from build123d import *

# Parameters (mm, degrees)
SKETCH_R    = 1.6
SKETCH_R_2  = 2.6
PAD_DEPTH   = 3
FILLET_R    = 3
FILLET001_R = 3
FILLET002_R = 3
FILLET003_R = 3
FILLET004_R = 3


with BuildPart() as part:
    # Sketch → Pad (new body)
    with BuildSketch(Plane.XY):
        Polygon((3, 50), (13, 50), (13, 37), (20, 37), (20, 23), (13, 23), (13, -20), (3, -20), (3, -7), (-4, -7), (-4, 7), (3, 7), align=None)
        Circle(SKETCH_R, mode=Mode.SUBTRACT)
        with Locations((16, 30)):
            Circle(SKETCH_R, mode=Mode.SUBTRACT)
        with Locations((8, 45)):
            Circle(SKETCH_R_2, mode=Mode.SUBTRACT)
        with Locations((8, -15)):
            Circle(SKETCH_R_2, mode=Mode.SUBTRACT)
    extrude(amount=PAD_DEPTH)

    # Fillet
    fillet_edges = [part.edges().sort_by_distance(p)[0] for p in [
        (13, -20, 1.5),
        (3, -20, 1.5),
        (20, 23, 1.5),
        (20, 37, 1.5),
        (-4, -7, 1.5),
        (-4, 7, 1.5),
        (3, 50, 1.5),
        (13, 50, 1.5),
    ]]
    fillet(fillet_edges, radius=FILLET_R)

    # Fillet001
    fillet001_edges = [part.edges().sort_by_distance(p)[0] for p in [
        (13, 37, 1.5),
    ]]
    fillet(fillet001_edges, radius=FILLET001_R)

    # Fillet002
    fillet002_edges = [part.edges().sort_by_distance(p)[0] for p in [
        (13, 23, 1.5),
    ]]
    fillet(fillet002_edges, radius=FILLET002_R)

    # Fillet003
    fillet003_edges = [part.edges().sort_by_distance(p)[0] for p in [
        (3, -7, 1.5),
    ]]
    fillet(fillet003_edges, radius=FILLET003_R)

    # Fillet004
    fillet004_edges = [part.edges().sort_by_distance(p)[0] for p in [
        (3, 7, 1.5),
    ]]
    fillet(fillet004_edges, radius=FILLET004_R)


solid = part.part
Check sheet for the modelled part. Datum: model origin and axes. Units: mm. A direction names the side the tool comes from. Give positions to 0.01 mm unless a question says otherwise; leave off trailing zeros. Loops run counter-clockwise (first coordinate to the right, second up) from the corner with the lowest first, then second, coordinate; pieces in that order, holes last. Notation, with made-up numbers: M 55,3.25 L 70,3.25 A33 ccw 70,40.25 Z; hole C 41.25,-40 d6. An arc over 180 degrees is marked long. Use a Markdown table: item, result. Add a question column.
Q1. Scan lines: line 1 along Y through (x, z) = (8, 1.2); line 2 along Y through (x, z) = (6.75, 1.95); line 3 along X through (y, z) = (-2.5, 0.4). Record each from-to range of solid material in increasing order. Write a range as [from, to].
Q2. Sectioned sample at C-C, the plane z = 0.75. Record the cut outline in (x, y).
Q3. Sectioned sample at D-D, the plane y = 45. Record the cut outline in (x, z), then the cut area to 3 significant figures.
Q4. Tool access check on faces 4 (the flat face through (3, -14, 1)), 5 (the flat face through (13, 2, 1)), 6 (the flat face through (8, 50, 1)). Record the directions out of +Z, -Z, +X, -X, +Y, -Y that give a thin tool (end or side, any length) a straight path to the whole face; none if there is none.
Q5. Mould release check, pull along X, two halves, no side actions. Record for faces 1 (the flat face through (13, 44, 1)), 2 (the cylindrical face through (10.4, -16, 1.5)), 3 (the cylindrical face through (2.14, -7.9, 1.52)): pulls with the +X half, pulls with the -X half, needs draft (parallel to the pull), parting line crosses it, or undercut.
Q6. Sectioned sample at A-A, the plane x = 8. Record the cut outline in (y, z), then the cut area to 3 significant figures.
Q7. Go/stop test with flat-tipped pins: pin 1 (10 mm diameter, centred on x = 13.5, y = 29.5, fed in from -Z); pin 2 (1.1 mm diameter, centred on x = 16.5, z = 1.5, fed in from +Y); pin 3 (1.5 mm diameter, centred on y = 30.5, z = 2, fed in from -X); pin 4 (1.1 mm diameter, centred on x = -0.5, z = 1.5, fed in from +Y). Record where each tip stops, or that it passes through.
Q8. Sectioned sample at B-B, the plane y = 0. Record the cut outline in (x, z).
Verdict:
| question | item | result |
|---|---|---|
| 1 | line 1 | [-20, -17.6], [-12.4, 42.4], [47.6, 50] |
| 1 | line 2 | [-20, -17.28], [-12.72, 42.72], [47.28, 50] |
| 1 | line 3 | [-4, 13] |
| 2 | outline | M -4,-4 A3 ccw -1,-7 L 0,-7 A3 cw 3,-10 L 3,-17 A3 ccw 6,-20 L 10,-20 A3 ccw 13,-17 L 13,20 A3 cw 16,23 L 17,23 A3 ccw 20,26 L 20,34 A3 ccw 17,37 L 16,37 A3 cw 13,40 L 13,47 A3 ccw 10,50 L 6,50 A3 ccw 3,47 L 3,10 A3 cw 0,7 L -1,7 A3 ccw -4,4 Z; hole C 0,0 d3.2; hole C 8,-15 d5.2; hole C 8,45 d5.2; hole C 16,30 d3.2 |
| 3 | outline | M 3,0 L 5.4,0 L 5.4,3 L 3,3 Z; M 10.6,0 L 13,0 L 13,3 L 10.6,3 Z |
| 3 | area | 14.4 mm^2 |
| 4 | face 4 | +Z, -Z, -X, -Y |
| 4 | face 5 | +Z, -Z, +X, -Y |
| 4 | face 6 | +Z, -Z, +X, -X, +Y |
| 5 | face 1 | pulls with the +X half |
| 5 | face 2 | undercut |
| 5 | face 3 | pulls with the -X half |
| 6 | outline | M -20,0 L -17.6,0 L -17.6,3 L -20,3 Z; M -12.4,0 L 42.4,0 L 42.4,3 L -12.4,3 Z; M 47.6,0 L 50,0 L 50,3 L 47.6,3 Z |
| 6 | area | 179 mm^2 |
| 7 | pin 1 | z = 0 |
| 7 | pin 2 | y = 37 |
| 7 | pin 3 | x = 3 |
| 7 | pin 4 | y = 7 |
| 8 | outline | M -4,0 L -1.6,0 L -1.6,3 L -4,3 Z; M 1.6,0 L 13,0 L 13,3 L 1.6,3 Z |
